Can you work these out from the drawing? Everything is in mm from the part's minimum corner. A direction names the side the tool comes from. Give positions to 0.01 mm unless a question says otherwise; leave off trailing zeros. Write each loop counter-clockwise with the first axis right and the second up, starting at its lowest first coordinate (ties: lowest second). Pieces come first, ordered by that corner, then holes. Notation, with made-up numbers: (66, 80) - (95, 80) arc R17 cw to (95, 92) - close; hole circle Ø7 at (-13, 23). An arc over 180 degrees is marked (long way). Write each question's results on one line, items separated by ' | '. Start each with the question number.
Item 1: Suppose I cut it at B-B on x = 10. List the corners of the cut face in (y, z) for me, then the cut area to 3 significant figures.
Item 2: Suppose I cut it at C-C on y = 16.25. List the corners of the cut face in (x, z) for me.
Item 3: Please list where these lines run through material, in increasing order: line 1 along Y through (x, z) = (10, 0.7); line 2 along X through (y, z) = (15, 1.35); line 3 along X through (y, z) = (4.75, 3.45) (1 decimal).
Item 4: We'd pull the mould along Y, two halves only. Please class the marked faces 1, 2 and 3: +Y half, -Y half, draft (parallel to the pull), parting line (faces both ways), or undercut.
Item 5: Suppose I cut it at D-D on z = 4.55. Count the separate pieces of the cut face and the enclosed holes in it, then the cut area to 3 significant figures.
Item 6: Which directions (+Z, -Z, +X, -X, +Y, -Y) give clear straight access to the entire face, cutting with the end or side of a thin tool? Please do the marked faces 4 and 5.
Item 7: Will this pin go through, and if not, where does the flat tip stop? P1, Ø5, axis at x = 10, y = 15, coming from the +Z side.
Item 8: Suppose I cut it at A-A on z = 1.8. List the corners of the cut face in (x, y) for me.
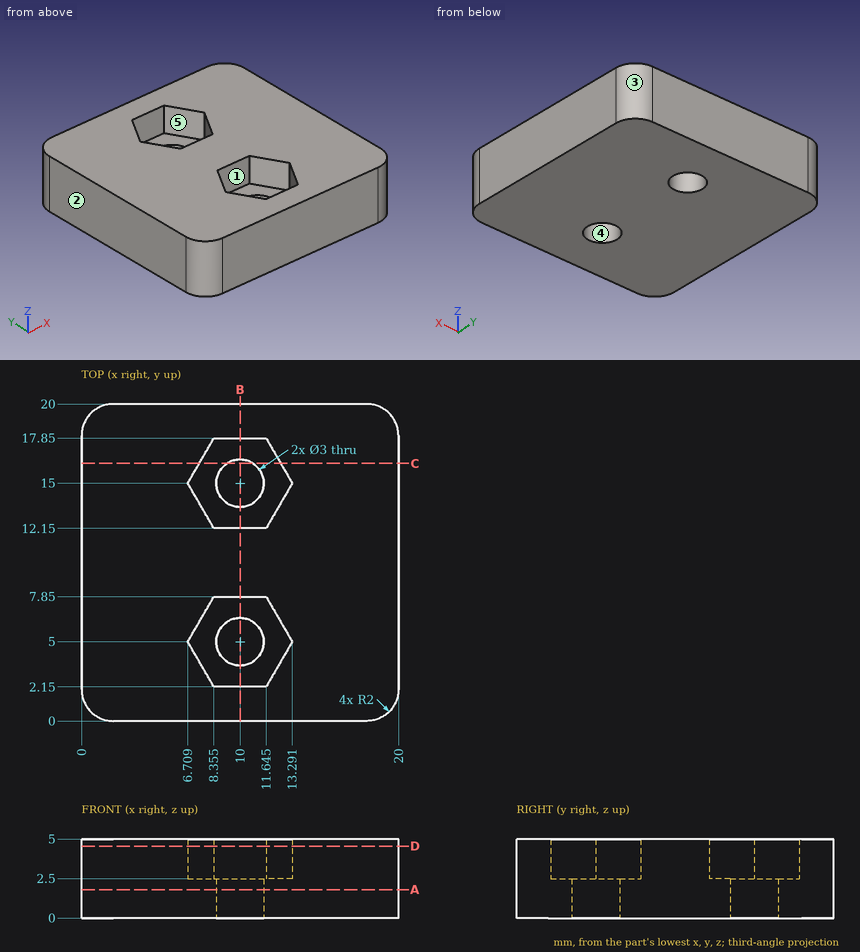
Checked values:
1) outline: (0, 0) - (3.5, 0) - (3.5, 2.5) - (2.15, 2.5) - (2.15, 5) - (0, 5) - close; (6.5, 0) - (13.5, 0) - (13.5, 2.5) - (12.15, 2.5) - (12.15, 5) - (7.85, 5) - (7.85, 2.5) - (6.5, 2.5) - close; (16.5, 0) - (20, 0) - (20, 5) - (17.85, 5) - (17.85, 2.5) - (16.5, 2.5) - close | area: 56.5 mm^2
2) outline: (0, 0) - (9.17, 0) - (9.17, 2.5) - (7.43, 2.5) - (7.43, 5) - (0, 5) - close; (10.83, 0) - (20, 0) - (20, 5) - (12.57, 5) - (12.57, 2.5) - (10.83, 2.5) - close
3) line 1: y = 0 to 3.5, 6.5 to 13.5, 16.5 to 20 | line 2: x = 0 to 8.5, 11.5 to 20 | line 3: x = 0 to 6.9, 13.1 to 20
4) face 1: undercut | face 2: draft | face 3: +Y half
5) separate pieces: 1 | enclosed holes: 2 | area: 340 mm^2
6) face 4: +Z, -Z | face 5: +Z
7) P1: stops at z = 2.5
8) outline: (0, 2) arc R2 ccw to (2, 0) - (18, 0) arc R2 ccw to (20, 2) - (20, 18) arc R2 ccw to (18, 20) - (2, 20) arc R2 ccw to (0, 18) - close; hole circle Ø3 at (10, 5); hole circle Ø3 at (10, 15)
